Autodesk Fusion 360 part; units mm, degrees
sketch "Sketch1" plane through (0, 0, 0) normal (0, 1, 0) x (1, 0, 0)
  circle A0 centre (-85.0015, -22.7761) radius 10.5
  circle A1 centre (-85.0015, 22.7761) radius 10.5
  line L0 (-71.2336, 33.2168) -> (-86.0563, 40.1287)
  line L1 (-77.1365, 6.7486) -> (-94.5913, 8.2757)
  line L2 (-77.1374, -6.7486) -> (-94.5913, -8.2757)
  line L3 (-71.2336, -33.2168) -> (-86.0563, -40.1287)
  line L4 (-69.5015, 22.7761) -> (-69.5015, -22.7761)
  line L5 (-69.5015, 22.7761) -> (-69.5015, 30.4979)
  line L6 (-69.5015, -22.7761) -> (-69.5015, -30.4979)
  line L7 (-74.398, 3.7596) -> (-74.3988, -3.7604)
  arc A2 (-97.8481, 5.454) -> (-97.8481, -5.454) centre (0, 0) ccw
  arc A3 (-69.5015, 30.4979) -> (-71.2336, 33.2168) centre (-72.5015, 30.4979) ccw
  arc A4 (-87.466, 44.2007) -> (-86.0563, 40.1287) centre (-84.7884, 42.8476) ccw
  arc A5 (-94.5913, 8.2757) -> (-97.8481, 5.454) centre (-94.8528, 5.2871) ccw
  arc A6 (-97.8481, -5.454) -> (-94.5913, -8.2757) centre (-94.8528, -5.2871) ccw
  arc A7 (-77.1374, -6.7486) -> (-74.3988, -3.7604) centre (-77.3988, -3.7601) ccw
  arc A8 (-74.398, 3.7596) -> (-77.1365, 6.7486) centre (-77.398, 3.76) ccw
  arc A9 (-71.2336, -33.2168) -> (-69.5015, -30.4979) centre (-72.5015, -30.4979) ccw
  arc A10 (-86.0563, -40.1287) -> (-87.466, -44.2007) centre (-84.7884, -42.8476) ccw
  arc A11 (-46.4263, 94.1785) -> (46.4263, 94.1785) centre (0, 0) ccw
  arc A12 (-43.2519, 93.8511) -> (-46.4263, 94.1785) centre (-45.0998, 91.4877) ccw
  line L8 (-9.7255, 67.6367) -> (-43.2519, 93.8511)
  line L9 (7.8776, 67) -> (-7.8776, 67)
  line L10 (43.2519, 93.8511) -> (9.7255, 67.6367)
  arc A13 (46.4263, 94.1785) -> (43.2519, 93.8511) centre (45.0998, 91.4877) ccw
  arc A14 (-9.7255, 67.6367) -> (-7.8776, 67) centre (-7.8776, 70) ccw
  arc A15 (7.8776, 67) -> (9.7255, 67.6367) centre (7.8776, 70) ccw
  arc A16 (-46.4263, 94.1785) -> (46.4263, 94.1785) centre (0, 0) ccw
  arc A17 (-9.7255, 67.6367) -> (-7.8776, 67) centre (-7.8776, 70) ccw
  circle A18 centre (100.6317, 13.2484) radius 1.5
  circle A19 centre (-100.6317, 13.2484) radius 1.5
  circle A20 centre (-34.715, -95.3788) radius 1.5
  circle A21 centre (34.715, -95.3788) radius 1.5
  circle A22 centre (-44.8298, 89.3777) radius 1.55
  circle A23 centre (44.8298, 89.3777) radius 1.55
  line L11 (41.8995, 83.9078) -> (14.0372, 62.1222)
  arc A24 (7.8776, 60) -> (14.0372, 62.1222) centre (7.8776, 70) ccw
  line L12 (7.8776, 60) -> (-7.8776, 60)
  arc A25 (-14.0372, 62.1222) -> (-7.8776, 60) centre (-7.8776, 70) ccw
  line L13 (-14.0372, 62.1222) -> (-41.8995, 83.9078)
  arc A26 (-49.766, 84.4236) -> (-87.466, 44.2007) centre (0, 0) ccw
  arc A27 (-87.466, -44.2007) -> (49.766, 84.4236) centre (0, 0) ccw
  arc A28 (-41.8995, 83.9078) -> (-49.766, 84.4236) centre (-46.2112, 78.3934) ccw
  arc A29 (49.766, 84.4236) -> (41.8995, 83.9078) centre (46.2112, 78.3934) ccw
  dimension "d83" = 3
  dimension "d84" = 3
  dimension "d96" = 3
  dimension "d97" = 3
extrude "Extrude1" add sketch "Sketch1" along normal blind 2
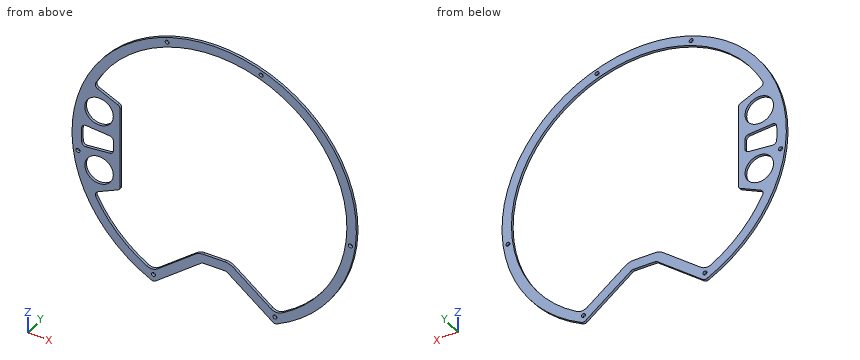
Read the model definition and answer for the solid it produces. Units are mm, in the model's axes. Round coordinates to 2 decimals unless told otherwise and drop trailing zeros. Order: outer loops, then holes, each group sorted by start corner. A loop starts at its lowest first (then second) coordinate and runs counter-clockwise, first axis right, second up. Notation, with made-up numbers: (-29.75, 33) - (20.25, 33) arc R6 cw to (20.25, 41) - close; hole circle Ø6 at (71, 14). An arc over 180 degrees is marked (long way). Use one line per item in the form item = value. Start each with the question number.
(1) The part is cut by section C-C (z = 0). Give the vertices of the cut face in (x, y).
(2) The part is cut by section D-D (x = 92.5). Give the vertices of the cut face in (y, z).
(3) The part is cut by section B-B (z = -70). Give the vertices of the cut face in (x, y).
(4) The part is cut by section A-A (x = 0). Give the vertices of the cut face in (y, z).
(5) Flat-ended cylindrical pins translate along their axes: pin 1 Ø2.5 at (x, z) = (-100.63, -13.25) entering from +Y; pin 2 Ø0.6 at (y, z) = (1, 11.5) entering from +X; pin 3 Ø1 at (x, y) = (-54.5, 1) entering from -Z; pin 4 Ø1 at (x, y) = (-40.5, 2) entering from +Z. Find the tip coordinate at first contact, or state that the pin passes through.
(6) Find the intervals of material crossed by line 1 along X through (y, z) = (1.85, 5); line 2 along Z through (x, y) = (-93.5, 1.45); line 3 along Z through (x, y) = (-73, 0.8), in increasing order. Write a range as from..to.
Checked values:
q1.outline = (-105, 0) - (-98, 0) - (-98, 2) - (-105, 2) - close; (-74.4, 0) - (-69.5, 0) - (-69.5, 2) - (-74.4, 2) - close; (98, 0) - (105, 0) - (105, 2) - (98, 2) - close
q2.outline = (0, -49.69) - (2, -49.69) - (2, -32.37) - (0, -32.37) - close; (0, 32.37) - (2, 32.37) - (2, 49.69) - (0, 49.69) - close
q3.outline = (-78.26, 0) - (-68.59, 0) - (-68.59, 2) - (-78.26, 2) - close; (-24.11, 0) - (-12.75, 0) - (-12.75, 2) - (-24.11, 2) - close; (12.75, 0) - (24.11, 0) - (24.11, 2) - (12.75, 2) - close; (68.59, 0) - (78.26, 0) - (78.26, 2) - (68.59, 2) - close
q4.outline = (0, -67) - (2, -67) - (2, -60) - (0, -60) - close; (0, 98) - (2, 98) - (2, 105) - (0, 105) - close
q5.pin_1 = through
q5.pin_2 = 104.4
q5.pin_3 = -90.05
q5.pin_4 = 97.08
q6.line_1 = -104.88..-97.87, -74.67..-69.5, 97.87..104.88
q6.line_2 = -47.78..-28.94, -16.61..-8.18, 8.18..16.61, 28.94..47.78
q6.line_3 = -75.47..-65.38, -34.04..34.04, 65.38..75.47
